Could you check a few things on this model? Use its own coordinates, in mm. A direction names the side the tool comes from. Give positions to 0.01 mm unless a question says otherwise; leave off trailing zeros. Loops run counter-clockwise (first coordinate to the right, second up) from the corner with the lowest first, then second, coordinate; pieces in that order, holes last. Notation, with made-up numbers: (16.5, -34) - (20.5, -34) arc R20 ccw to (20.5, -5) - close; hole circle Ø2 at (51, 2.5). An arc over 180 degrees is marked (long way). Use CSV: the item, a comma, the result in double quotes.
from build123d import *

# Parameters (mm, degrees)
F0_W      = 45
F0_H      = 45
F1_DEPTH  = 30
F2_SIZE   = 3
F4_D      = 5
F6_DEPTH  = 20
F7_R      = 9
F8_DEPTH  = 5
F10_D     = 10
F10_DEPTH = 30
F10_TIP   = 3.0043030951
F11_R     = 15
F12_DEPTH = 20
F13_R     = 1
F15_D     = 8.5


with BuildPart() as f1:
    # F0 (on Top) → F1 (new body)
    with BuildSketch(Plane.XY):
        with Locations((-22.5, -22.5)):
            Rectangle(F0_W, F0_H)
    extrude(amount=F1_DEPTH)

    # F2
    f2_edges = [f1.edges().sort_by_distance(p)[0] for p in [
        (-45, -45, 15),
        (0, -45, 15),
        (0, 0, 15),
        (-45, 0, 15),
    ]]
    chamfer(f2_edges, length=F2_SIZE)

    # F4 (through all)
    with Locations(Plane.XY.offset(30)):
        with Locations((-40.5312229203, -40.5312229203), (-40.5312229203, -4.4687770797), (-4.4687770797, -4.4687770797), (-4.4687770797, -40.5312229203)):
            Hole(F4_D / 2)

    # F5 (on face) → F6 (join)
    with BuildSketch(Plane.YZ):
        with BuildLine():
            ThreePointArc((-15.3121332332, 12.8588387864), (-15.0784435342, 13.9181036905), (-15, 15))
            ThreePointArc((-15, 15), (-15.2293520832, 16.8405648237), (-15.903381032, 18.5685596803))
            ThreePointArc((-15.903381032, 18.5685596803), (-17.7711474831, 20.8213360901), (-20.3588389028, 22.1878668015))
            ThreePointArc((-20.3588389028, 22.1878668015), (-23.2725024385, 22.4601099176), (-26.0685594955, 21.5966190679))
            ThreePointArc((-26.0685594955, 21.5966190679), (-28.3213359619, 19.7288526747), (-29.6878667454, 17.1411612856))
            ThreePointArc((-29.6878667454, 17.1411612856), (-29.9601099219, 14.2274976035), (-29.0966190145, 11.4314404058))
            ThreePointArc((-29.0966190145, 11.4314404058), (-27.2288526423, 9.1786640118), (-24.6411613131, 7.8121332628))
            ThreePointArc((-24.6411613131, 7.8121332628), (-21.7274976178, 7.5398900766), (-18.9314404058, 8.4033809855))
            ThreePointArc((-18.9314404058, 8.4033809855), (-16.6786639791, 10.271147398), (-15.3121332332, 12.8588387864))
        make_face()
        with BuildLine():
            ThreePointArc((-15.903381032, 18.5685596803), (-15.2293520832, 16.8405648237), (-15, 15))
            ThreePointArc((-15, 15), (-15.0784435342, 13.9181036905), (-15.3121332332, 12.8588387864))
            Line((-15.3121332332, 12.8588387864), (-14.4252352272, 15.8361507619))
            Line((-14.4252352272, 15.8361507619), (-15.903381032, 18.5685596803))
        make_face()
        with BuildLine():
            ThreePointArc((-20.3588389028, 22.1878668015), (-17.7711474831, 20.8213360901), (-15.903381032, 18.5685596803))
            Line((-15.903381032, 18.5685596803), (-17.3815269465, 21.3009688012))
            Line((-17.3815269465, 21.3009688012), (-20.3588389028, 22.1878668015))
        make_face()
        with BuildLine():
            Line((-16.1990311988, 9.8815269465), (-15.3121332332, 12.8588387864))
            ThreePointArc((-15.3121332332, 12.8588387864), (-16.6786639791, 10.271147398), (-18.9314404058, 8.4033809855))
            Line((-18.9314404058, 8.4033809855), (-16.1990311988, 9.8815269465))
        make_face()
        with BuildLine():
            ThreePointArc((-26.0685594955, 21.5966190679), (-23.2725024385, 22.4601099176), (-20.3588389028, 22.1878668015))
            Line((-20.3588389028, 22.1878668015), (-23.3361507619, 23.0747647728))
            Line((-23.3361507619, 23.0747647728), (-26.0685594955, 21.5966190679))
        make_face()
        with BuildLine():
            Line((-21.6638492381, 6.9252352272), (-18.9314404058, 8.4033809855))
            ThreePointArc((-18.9314404058, 8.4033809855), (-21.7274976178, 7.5398900766), (-24.6411613131, 7.8121332628))
            Line((-24.6411613131, 7.8121332628), (-21.6638492381, 6.9252352272))
        make_face()
        with BuildLine():
            ThreePointArc((-29.6878667454, 17.1411612856), (-28.3213359619, 19.7288526747), (-26.0685594955, 21.5966190679))
            Line((-26.0685594955, 21.5966190679), (-28.8009688012, 20.1184730535))
            Line((-28.8009688012, 20.1184730535), (-29.6878667454, 17.1411612856))
        make_face()
        with BuildLine():
            Line((-27.6184730535, 8.6990311988), (-24.6411613131, 7.8121332628))
            ThreePointArc((-24.6411613131, 7.8121332628), (-27.2288526423, 9.1786640118), (-29.0966190145, 11.4314404058))
            Line((-29.0966190145, 11.4314404058), (-27.6184730535, 8.6990311988))
        make_face()
        with BuildLine():
            ThreePointArc((-29.0966190145, 11.4314404058), (-29.9601099219, 14.2274976035), (-29.6878667454, 17.1411612856))
            Line((-29.6878667454, 17.1411612856), (-30.5747647728, 14.1638492381))
            Line((-30.5747647728, 14.1638492381), (-29.0966190145, 11.4314404058))
        make_face()
    extrude(amount=F6_DEPTH)

    # F7 (on face) → F8 (join)
    with BuildSketch(Plane.YZ.offset(20)):
        with Locations((-22.5, 15)):
            Circle(F7_R)
        Polygon((-29.687866787, 17.1411611458), (-22.5, 15), (-24.6411611458, 7.812133213), align=None, mode=Mode.SUBTRACT)
        Polygon((-24.6411611458, 7.812133213), (-22.5, 15), (-29.687866787, 17.1411611458), align=None)
    extrude(amount=F8_DEPTH)

    # F10
    with Locations(Plane.YZ.offset(25)):
        with Locations((-22.5, 15)):
            Hole(F10_D / 2, depth=F10_DEPTH)
            with Locations((0, 0, -(F10_DEPTH + F10_TIP / 2))):  # 118° drill point
                Cone(0, F10_D / 2, F10_TIP, mode=Mode.SUBTRACT)

    # F11 (on face) → F12 (join)
    with BuildSketch(Plane.XY.offset(30)):
        with Locations((-22.5, -22.5)):
            Circle(F11_R)
    extrude(amount=F12_DEPTH)

    # F13
    f13_edges = [f1.edges().sort_by_distance(p)[0] for p in [
        (-37.5, -22.5, 50),
    ]]
    fillet(f13_edges, radius=F13_R)

    # F15 (through all)
    with Locations(Plane.XY.offset(50)):
        with Locations((-22.5, -22.5)):
            Hole(F15_D / 2)


solid = f1.part
1) Suppose I cut it at D-D (z = 35.5). Please give me the cut outline in (x, y), plus the area to 3 significant figures.
Answer below:
outline,"circle Ø30 at (-22.5, -22.5); hole circle Ø8.5 at (-22.5, -22.5)"
area,"650 mm2"
2) Suppose I cut it at A-A (x = -22.5). Please give me the cut outline in (y, z), plus the area to 3 significant figures.
Answer below:
outline,"(-45, 0) - (-26.75, 0) - (-26.75, 50) - (-36.5, 50) arc R1 ccw to (-37.5, 49) - (-37.5, 30) - (-45, 30) - close; (-18.25, 0) - (0, 0) - (0, 30) - (-7.5, 30) - (-7.5, 49) arc R1 ccw to (-8.5, 50) - (-18.25, 50) - close"
area,"1,520 mm2"
3) Which directions (+Z, -Z, +X, -X, +Y, -Y) give clear straight access to the entire face, cutting with the end or side of a thin tool? Please do faces 1 (the cylindrical face through (22.465, -13.916, 17.703)), 2 (the flat face through (9.86, -29.117, 11.47)), 3 (the flat face through (20, -29, 10)), 4 (the cylindrical face through (-25.752, -37.143, 39.367)).
Answer below:
face 1,"+X"
face 2,"-Z, -Y"
face 3,"none"
face 4,"+Z"
4) I need wall thicknesses on line 1 along X through (y, z) = (-40, 23.5); line 2 along X through (y, z) = (-29, 4.5); line 3 along X through (y, z) = (-6.5, 22.5). Which ranges of each line are inside material? Lowest first, please.
Answer below:
line 1,"x = -45 to -42.97, -38.09 to -6.91, -2.03 to 0"
line 2,"x = -45 to 0"
line 3,"x = -45 to -41.99, -39.07 to -5.93, -3.01 to 0"
5) Suppose I cut it at B-B (x = 17). Please give me the cut outline in (y, z).
Answer below:
outline,"(-30.57, 14.16) - (-27.62, 8.7) - (-21.66, 6.93) - (-16.2, 9.88) - (-14.43, 15.84) - (-17.38, 21.3) - (-23.34, 23.07) - (-28.8, 20.12) - close; hole circle Ø10 at (-22.5, 15)"
6) I'm going to push flat-ended pins straight in: P1, Ø6.5, axis at x = -4.47, y = -4.47, coming from the +Z side; P2, Ø4, axis at x = -4.47, y = -40.53, coming from the +Z side; P3, Ø10, axis at x = 6, y = -18, coming from the -Z side; P4, Ø3, axis at x = 14, y = -20.5, coming from the +Z side. Where does each tip first touch, or does it pass through?
Answer below:
P1,"stops at z = 30"
P2,"passes through"
P3,"stops at z = 6.93"
P4,"stops at z = 22.68"
7) We'd pull the mould along Y, two halves only. Please class faces 5 (the flat face through (-25.81, -25.42, 50)), 6 (the cylindrical face through (-3.93, -6.91, 14.79)), 7 (the conical face through (-7.483, -22.613, 15.861)), 8 (the flat face through (-2, -1, 15)): +Y half, -Y half, draft (parallel to the pull), parting line (faces both ways), or undercut.
Answer below:
face 5,"draft"
face 6,"undercut"
face 7,"undercut"
face 8,"+Y half"
8) Suppose I cut it at C-C (y = -39). Please give me the cut outline in (x, z).
Answer below:
outline,"(-45, 0) - (-42.51, 0) - (-42.51, 30) - (-45, 30) - close; (-38.56, 0) - (-6.44, 0) - (-6.44, 30) - (-38.56, 30) - close; (-2.49, 0) - (0, 0) - (0, 30) - (-2.49, 30) - close"
